Model file for the job. Use its own axes, mm. Face numbers are marked on the shaded views. A direction names the side the tool comes from. Coordinates: 2 decimals unless noted, no trailing zeros. Write each loop counter-clockwise with the first axis right and the second up, starting at its lowest first coordinate (ties: lowest second). Pieces come first, ordered by that corner, then holes. Notation, with made-up numbers: (74, 11.5) - (99, 11.5) arc R18 ccw to (99, 20.5) - close; hole circle Ø4 at (17.5, 21.5). An arc over 180 degrees is marked (long way). Put each result on its own line as item: value. Start each with the question number.
1. Saw through at D-D, the plane y = 63. Write the cut outline in (x, z).
2. Drill centre lines: L1, parallel to Y at x = 12.7, z = 1.4; L2, parallel to X at y = 35.5, z = 7. Where is each one in solid material? Low to high. Write a range as from..to.
3. Drop a flat-ended pin along its axis: P1, Ø4.5, axis at x = 12.7, y = 138.27, coming from the +Z side. Give the stop position or say it passes through.
4. Saw through at A-A, the plane z = 17.25. Write the cut outline in (x, y).
5. Pull direction X, two halves, no side cores. Call the marked faces 1, 2 and 3: released by +X, released by -X, zero draft, split by the parting line, or undercut.
6. Saw through at B-B, the plane x = 4. Write the cut outline in (y, z).
7. Which spindle directions (+Z, -Z, +X, -X, +Y, -Y) get a long thin tool onto all of the face, cutting with end or side? Do the marked faces 4 and 5. Say none if no direction does.
8. Saw through at C-C, the plane y = 29.21. Write the cut outline in (x, z).
```python
from build123d import *

# Parameters (mm, degrees)
SKETCH1_W           = 25.4
SKETCH1_H           = 147.155789
BOSS_EXTRUDE1_DEPTH = 25.4
SKETCH2_W           = 20.32
SKETCH2_H           = 20.32
CUT_EXTRUDE1_DEPTH  = 148.155789
SKETCH3_R           = 2.4892
CUT_EXTRUDE2_DEPTH  = 26.4
SKETCH5_R           = 3.9624
CUT_EXTRUDE3_DEPTH  = 26.4


with BuildPart() as part:
    # Sketch1 → Boss-Extrude1 (new body)
    with BuildSketch(Plane.XY):
        with Locations((12.7, 73.5778945)):
            Rectangle(SKETCH1_W, SKETCH1_H)
    extrude(amount=BOSS_EXTRUDE1_DEPTH)

    # Sketch2 → Cut-Extrude1 (cut, through all)
    with BuildSketch(Plane(origin=(0, 147.155789, 0), x_dir=(1, 0, 0), z_dir=(0, 1, 0))):
        with Locations((12.7, -12.7)):
            Rectangle(SKETCH2_W, SKETCH2_H)
    extrude(amount=-CUT_EXTRUDE1_DEPTH, mode=Mode.SUBTRACT)

    # Sketch3 → Cut-Extrude2 (cut, through all)
    with BuildSketch(Plane(origin=(0, 0, 0), x_dir=(-1, 0, 0), z_dir=(0, 0, -1))):
        with Locations((-12.7, 138.265789)):
            Circle(SKETCH3_R)
        with Locations((-12.7, 117.945789)):
            Circle(SKETCH3_R)
        with Locations((-12.7, 29.21)):
            Circle(SKETCH3_R)
        with Locations((-12.7, 8.89)):
            Circle(SKETCH3_R)
    extrude(amount=-CUT_EXTRUDE2_DEPTH, mode=Mode.SUBTRACT)

    # Sketch5 → Cut-Extrude3 (cut, through all)
    with BuildSketch(Plane(origin=(25.4, 0, 0), x_dir=(0, 0, -1), z_dir=(1, 0, 0))):
        with Locations((-7.5184, 17.3804072)):
            Circle(SKETCH5_R)
    extrude(amount=-CUT_EXTRUDE3_DEPTH, mode=Mode.SUBTRACT)


solid = part.part
```
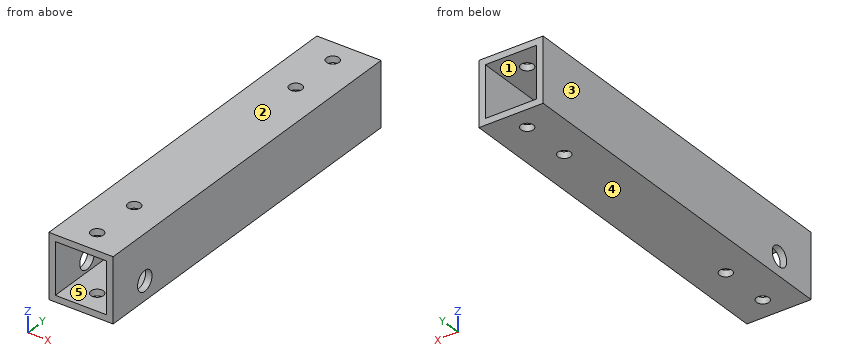
Final values:
1. outline: (0, 0) - (25.4, 0) - (25.4, 25.4) - (0, 25.4) - close; hole (2.54, 2.54) - (22.86, 2.54) - (22.86, 22.86) - (2.54, 22.86) - close
2. L1: y = 0..6.4, 11.38..26.72, 31.7..115.46, 120.43..135.78, 140.75..147.16
2. L2: x = 0..2.54, 22.86..25.4
3. P1: passes through
4. outline: (0, 0) - (2.54, 0) - (2.54, 147.16) - (0, 147.16) - close; (22.86, 0) - (25.4, 0) - (25.4, 147.16) - (22.86, 147.16) - close
5. face 1: undercut
5. face 2: zero draft
5. face 3: released by -X
6. outline: (0, 0) - (147.16, 0) - (147.16, 2.54) - (0, 2.54) - close; (0, 22.86) - (147.16, 22.86) - (147.16, 25.4) - (0, 25.4) - close
7. face 4: -Z, +X, -X, +Y, -Y
7. face 5: +Y, -Y
8. outline: (0, 0) - (10.21, 0) - (10.21, 2.54) - (2.54, 2.54) - (2.54, 22.86) - (10.21, 22.86) - (10.21, 25.4) - (0, 25.4) - close; (15.19, 0) - (25.4, 0) - (25.4, 25.4) - (15.19, 25.4) - (15.19, 22.86) - (22.86, 22.86) - (22.86, 2.54) - (15.19, 2.54) - close
